```python
from build123d import *

# Parameters (mm, degrees)
BASE_FLANGE1_DEPTH = 50
SKETCH3_R          = 2.5
EXTRUDE1_DEPTH     = 2
FILLET1_R          = 2


# Sheet-metal steps are written as plain solids
with BuildPart() as part:
    # Sketch1 → Base-Flange1 (new, symmetric)
    with BuildSketch(Plane(origin=(0, 0, 0), x_dir=(-1, 0, 0), z_dir=(0, 1, 0))):
        with BuildLine():
            Line((0, 0), (0, -8))
            ThreePointArc((0, -8), (-0.585786438, -9.414213562), (-2, -10))
            Line((-2, -10), (-8.5, -10))
            ThreePointArc((-8.5, -10), (-11.328427125, -11.171572875), (-12.5, -14))
            Line((-12.5, -14), (-12.5, -25))
            Line((-12.5, -25), (-10.5, -25))
            Line((-10.5, -25), (-10.5, -14))
            ThreePointArc((-10.5, -14), (-9.914213562, -12.585786438), (-8.5, -12))
            Line((-8.5, -12), (-2, -12))
            ThreePointArc((-2, -12), (0.828427125, -10.828427125), (2, -8))
            Line((2, -8), (2, 0))
            Line((2, 0), (0, 0))
        make_face()
    extrude(amount=BASE_FLANGE1_DEPTH, both=True)

    # Sketch3 → Extrude1 (cut)
    with BuildSketch(Plane(origin=(12.5, 0, 0), x_dir=(0, 0, 1), z_dir=(1, 0, 0))):
        with Locations((-19, 35)):
            Circle(SKETCH3_R)
        with Locations(Location((-19, -35, 0), (0, 0, 180))):
            Circle(SKETCH3_R)
    extrude(amount=-EXTRUDE1_DEPTH, mode=Mode.SUBTRACT)

    # Fillet1
    fillet1_edges = [part.edges().sort_by_distance(p)[0] for p in [
        (-1, -50, 0),
        (11.5, -50, -25),
        (-1, 50, 0),
        (11.5, 50, -25),
    ]]
    fillet(fillet1_edges, radius=FILLET1_R)


solid = part.part
```
The model under review builds one solid part; all positions refer to its coordinate system, in mm. A direction names the side the tool comes from. Give positions to 0.01 mm unless a question says otherwise; leave off trailing zeros. Write each loop counter-clockwise with the first axis right and the second up, starting at its lowest first coordinate (ties: lowest second). Pieces come first, ordered by that corner, then holes.
(1) Consider section B-B, the plane y = 35. Give the boundary of the cut face in (x, z).
(2) Consider section D-D, the plane z = -3. Give the boundary of the cut face in (x, y).
(3) The part is to be moulded in two halves that separate along Z. For faces 1 (the cylindrical face through (-0.99, 49.43, -0.6)), 2 (the flat face through (10.5, 1, -20)), 3 (the cylindrical face through (11.49, -49.43, -24.4)), 4 (the cylindrical face through (11.5, -35.1, -21.5)), say which applies: released by +Z, released by -Z, zero draft, split by the parting line, or undercut.
(4) To check wall thickness, follow L1, parallel to Y at x = 11.4, z = -19; L2, parallel to X at y = -13, z = -7.25; L3, parallel to X at y = 31, z = -16.5. State the ranges of each line that lie inside material, in increasing order.
(5) Consider section A-A, the plane z = -19. Give the boundary of the cut face in (x, y).
(6) Tool access review of faces 5 (the cylindrical face through (-0.99, -49.43, -0.6)), 6 (the flat face through (5, 1, -12)), 7 (the flat face through (0, 1, -4)): name each direction out of +Z, -Z, +X, -X, +Y, -Y from which nothing blocks a thin tool from reaching the whole face with its end or side.
(7) Consider section C-C, the plane y = -1.5. Give the boundary of the cut face in (x, z).
(8) For P1, Ø5, axis at x = 4.5, y = 15, coming from the -Z side; P2, Ø5.5, axis at y = -18.5, z = -17, coming from the -X side; P3, Ø5, axis at x = 7, y = 12.5, coming from the -Z side, all flat-tipped, find the tip position at first contact; note any pin that passes through.
Returned:
1. outline: (-2, -8) arc R4 ccw to (2, -12) - (8.5, -12) arc R2 cw to (10.5, -14) - (10.5, -16.5) - (12.5, -16.5) - (12.5, -14) arc R4 ccw to (8.5, -10) - (2, -10) arc R2 cw to (0, -8) - (0, 0) - (-2, 0) - close; (10.5, -25) - (12.5, -25) - (12.5, -21.5) - (10.5, -21.5) - close
2. outline: (-2, -50) - (0, -50) - (0, 50) - (-2, 50) - close
3. face 1: released by +Z
3. face 2: zero draft
3. face 3: released by -Z
3. face 4: undercut
4. L1: y = -50 to -37.5, -32.5 to 32.5, 37.5 to 50
4. L2: x = -2 to 0
4. L3: x = 10.5 to 12.5
5. outline: (10.5, -50) - (12.5, -50) - (12.5, -37.5) - (10.5, -37.5) - close; (10.5, -32.5) - (12.5, -32.5) - (12.5, 32.5) - (10.5, 32.5) - close; (10.5, 37.5) - (12.5, 37.5) - (12.5, 50) - (10.5, 50) - close
6. face 5: +Z, +X, -X, -Y
6. face 6: -Z, -X, +Y, -Y
6. face 7: +Z, +X, +Y, -Y
7. outline: (-2, -8) arc R4 ccw to (2, -12) - (8.5, -12) arc R2 cw to (10.5, -14) - (10.5, -25) - (12.5, -25) - (12.5, -14) arc R4 ccw to (8.5, -10) - (2, -10) arc R2 cw to (0, -8) - (0, 0) - (-2, 0) - close
8. P1: stops at z = -12
8. P2: stops at x = 10.5
8. P3: stops at z = -12.27
